Geometry: see drawing. Coordinates: mm, zero at the bounding-box minimum. Round coordinates to 2 decimals unless told otherwise and drop trailing zeros. Loops run counter-clockwise (first coordinate to the right, second up) from the corner with the lowest first, then second, coordinate; pieces in that order, holes last. Notation, with made-up numbers: (-14.75, 32.5) - (14.25, 32.5) arc R5 ccw to (14.25, 37.5) - close; hole circle Ø2 at (-25, -2.5). An arc over 180 degrees is marked (long way). Answer in a Markdown table with one row per item. Add a question column.
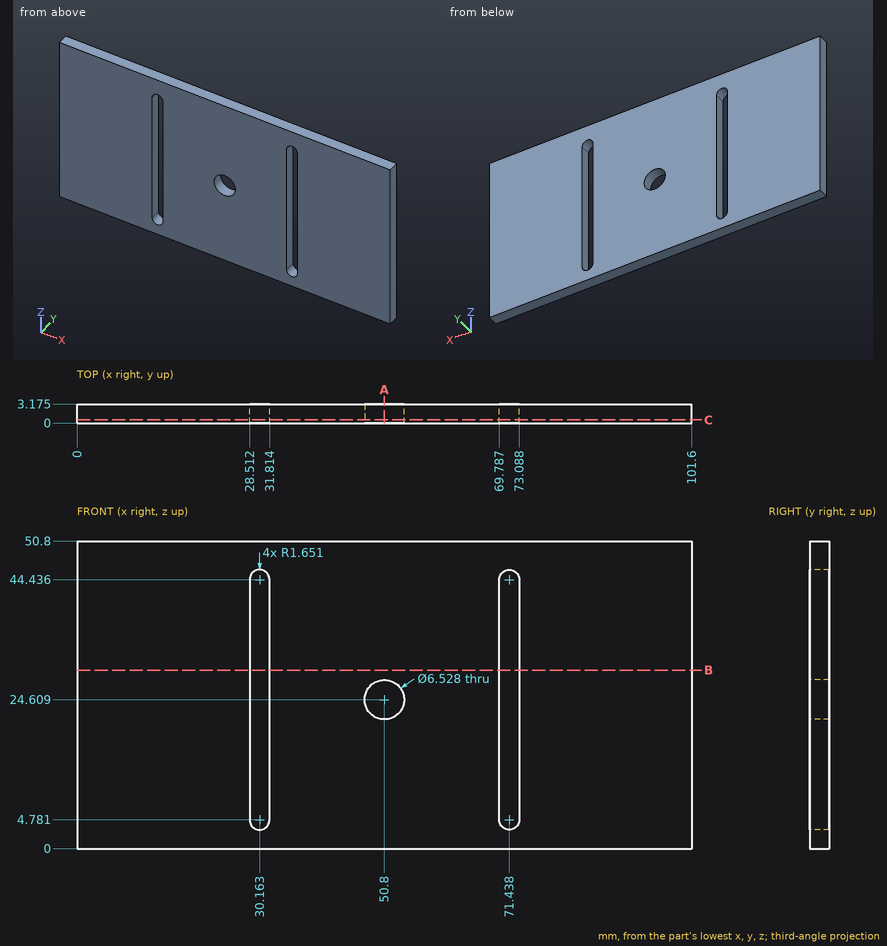
1) Section C-C, the plane y = 0.55. Return the cut outline in (x, z), and give its area (3 significant figures).
2) Section B-B, the plane z = 29.5. Return the cut outline in (x, y) (1 decimal).
3) Section A-A, the plane x = 50.8. Return the cut outline in (y, z) (1 decimal).
4) Material intervals for line 1 along X through (y, z) = (1.1, 9); line 2 along X through (y, z) = (0.85, 25.5) (1 decimal); line 3 along Z through (x, y) = (50.8, 1.8) (1 decimal), sorted ascending. Write a range as from..to.
Evaluation:
| question | item | result |
|---|---|---|
| 1 | outline | (0, 0) - (101.6, 0) - (101.6, 50.8) - (0, 50.8) - close; hole (28.51, 4.78) arc R1.65 ccw to (31.81, 4.78) - (31.81, 44.44) arc R1.65 ccw to (28.51, 44.44) - close; hole circle Ø6.53 at (50.8, 24.61); hole (69.79, 4.78) arc R1.65 ccw to (73.09, 4.78) - (73.09, 44.44) arc R1.65 ccw to (69.79, 44.44) - close |
| 1 | area | 4,850 mm² |
| 2 | outline | (0, 0) - (28.5, 0) - (28.5, 3.2) - (0, 3.2) - close; (31.8, 0) - (69.8, 0) - (69.8, 3.2) - (31.8, 3.2) - close; (73.1, 0) - (101.6, 0) - (101.6, 3.2) - (73.1, 3.2) - close |
| 3 | outline | (0, 0) - (3.2, 0) - (3.2, 21.3) - (0, 21.3) - close; (0, 27.9) - (3.2, 27.9) - (3.2, 50.8) - (0, 50.8) - close |
| 4 | line 1 | x = 0..28.51, 31.81..69.79, 73.09..101.6 |
| 4 | line 2 | x = 0..28.5, 31.8..47.7, 53.9..69.8, 73.1..101.6 |
| 4 | line 3 | z = 0..21.3, 27.9..50.8 |
